Here's the drawing with two shaded views (mm, measured from the low corner). I have some questions. Round coordinates to 2 decimals unless told otherwise and drop trailing zeros. Order: outer loops, then holes, each group sorted by start corner. A loop starts at its lowest first (then second) coordinate and runs counter-clockwise, first axis right, second up.
Q1. If we section it at D-D (x = 78): Please give me the cut outline in (y, z).
Q2. If I drill on line 1 (Y direction, x = 48.5, z = 5.25); line 2 (Y direction, x = 73, z = 6.25); line 3 (X direction, y = 57.5, z = 3.25), over which ranges is the centre line in solid material (lowest first)?
Q3. Will these pins go through, and if not, where does the flat tip stop? P1, Ø5, axis at x = 12.192, y = 89.027, coming from the +Z side; P2, Ø1.8, axis at x = 12.192, y = 133.223, coming from the +Z side.
Q4. If we section it at C-C (y = 102): Please give me the cut outline in (x, z) (1 decimal), plus the area to 3 significant figures.
Q5. If we section it at A-A (x = 67): Please give me the cut outline in (y, z).
Q6. We'd pull the mould along X, two halves only. Please class the marked faces 1, 2, 3 and 4: pulls with the +X half, pulls with the -X half, needs draft (parallel to the pull), parting line crosses it, or undercut.
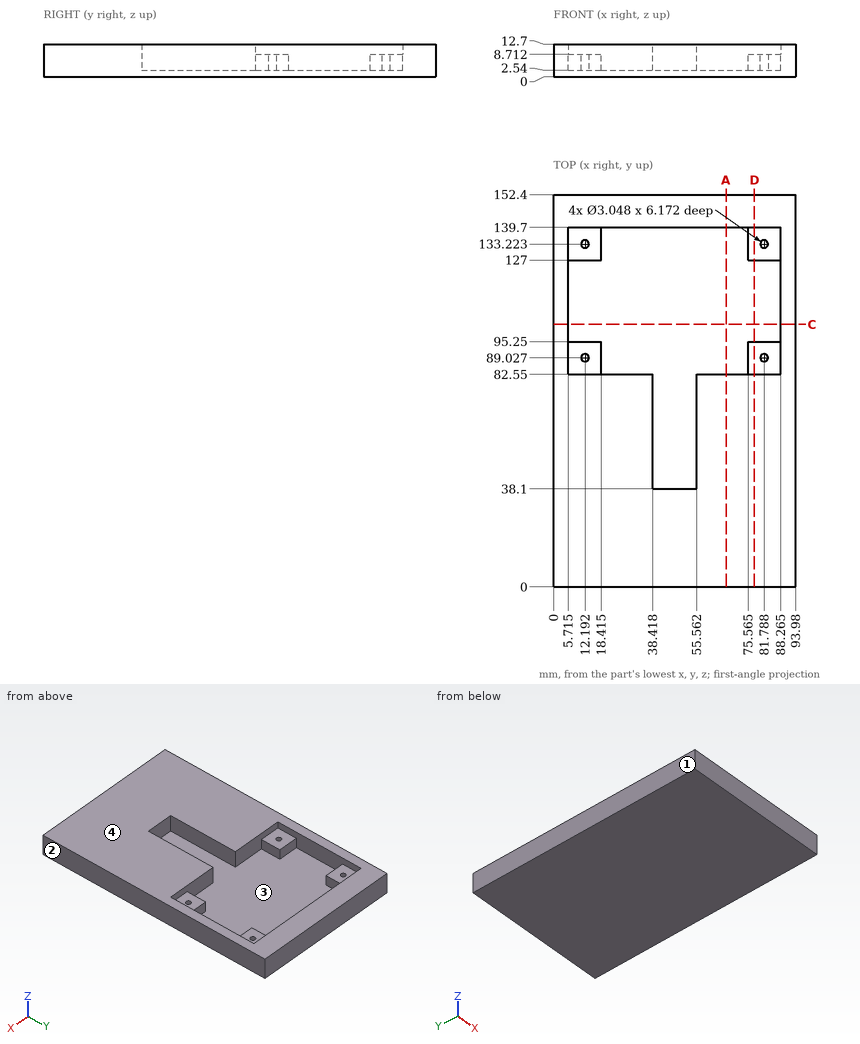
Solution:
1. outline: (0, 0) - (152.4, 0) - (152.4, 12.7) - (139.7, 12.7) - (139.7, 8.71) - (127, 8.71) - (127, 2.54) - (95.25, 2.54) - (95.25, 8.71) - (82.55, 8.71) - (82.55, 12.7) - (0, 12.7) - close
2. line 1: y = 0 to 38.1, 139.7 to 152.4
2. line 2: y = 0 to 82.55, 139.7 to 152.4
2. line 3: x = 0 to 38.42, 55.56 to 93.98
3. P1: stops at z = 8.71
3. P2: stops at z = 2.54
4. outline: (0, 0) - (94, 0) - (94, 12.7) - (88.3, 12.7) - (88.3, 2.5) - (5.7, 2.5) - (5.7, 12.7) - (0, 12.7) - close
4. area: 355 mm2
5. outline: (0, 0) - (152.4, 0) - (152.4, 12.7) - (139.7, 12.7) - (139.7, 2.54) - (82.55, 2.54) - (82.55, 12.7) - (0, 12.7) - close
6. face 1: pulls with the -X half
6. face 2: pulls with the +X half
6. face 3: undercut
6. face 4: needs draft
